Design review of the part built by this model. Coordinates are the model's own, in mm. A direction names the side the tool comes from. Coordinates: 2 decimals unless noted, no trailing zeros. Loops run counter-clockwise (first coordinate to the right, second up) from the corner with the lowest first, then second, coordinate; pieces in that order, holes last. Notation, with made-up numbers: (47.5, 46) - (59.5, 46) arc R17 ccw to (59.5, 56) - close; hole circle Ø9 at (82.25, 34.5). An arc over 180 degrees is marked (long way). Answer in a Markdown table with one row per item. Add a question column.
(1) Clearance check with flat-ended pins moving along their axes: pin 1 (0.8 mm diameter, centred on x = -4.5, z = 6.5, fed in from +Y); pin 2 (12 mm diameter, centred on y = 13, z = 15.5, fed in from +X); pin 3 (5.5 mm diameter, centred on y = 0, z = 5, fed in from -X). State where each tip first meets the part, or that it passes through.
(2) To check wall thickness, follow L1, parallel to Y at x = 0, z = 55.35; L2, parallel to X at y = -7, z = 55 (3 decimals); L3, parallel to Z at x = -3.5, y = -9.5. State the ranges of each line that lie inside material, in increasing order. Write a range as [from, to].
(3) For faces 5 (the face through (0, 4, 35)), 6 (the face through (6.428, 4.929, 23.493)), 7 (the face through (-5, 9, 54)), 8 (the face through (7.5, -1, 3)), list the 3-axis set-ups (+Z, -Z, +X, -X, +Y, -Y) from which the entire face can be reached by the end or side of a thin tool; tool diameter is ignored.
(4) We need section D-D, the plane y = 15. Write out the cut boundary in (x, z), plus the area to 3 significant figures.
(5) We need section B-B, the plane z = 5.5. Write out the cut boundary in (x, y).
(6) We need section C-C, the plane x = 0. Give the number of separate pieces and of enclosed holes in the cut face, plus the area to 3 significant figures.
(7) We need section A-A, the plane y = 0. Write out the cut boundary in (x, z), plus the area to 3 significant figures.
(8) The part is to be moulded in two halves that separate along Y. For faces 1 (the face through (-5, 4, 3)), 2 (the face through (-11.083, 8.101, 55.479)), 3 (the face through (-4.336, -19.524, 55.479)), 4 (the face through (0, -13, 55)), say which applies: released by +Y, released by -Y, zero draft, split by the parting line, or undercut.
from build123d import *

# Parameters (mm, degrees)
SKETCH_1_R               = 8.5
EXTRUDE_1_DEPTH          = 33
SKETCH_2_R               = 8.5
EXTRUDE_2_DEPTH          = 11
SKETCH_3_R               = 10
EXTRUDE_3_DEPTH          = 10
CHAMFER_2_SIZE           = 0.5
SKETCH_12_W              = 1
SKETCH_12_H              = 0.4
SKETCH_13_R              = 5
CUT_EXTRUDE_1_DEPTH      = 20
EXTRUDE_START            = 7.5
SKETCH_19_R              = 8.5
EXTRUDE_6_DEPTH          = 7.5
SKETCH_20_R              = 5
CUT_EXTRUDE_5_DEPTH      = 7.5
CUT_EXTRUDE_6_DEPTH      = 16.5
CUT_EXTRUDE_6_DEPTH_BACK = 16.5
SKETCH_21_R              = 1.5
SKETCH_14_R              = 20
SKETCH_14_R_2            = 2
EXTRUDE_7_DEPTH          = 3
EXTRUDE_START_2          = 7
SKETCH_23_R              = 5
EXTRUDE_8_DEPTH          = 7
CUT_EXTRUDE_START        = -44
SKETCH_24_R              = 5
CUT_EXTRUDE_7_DEPTH      = 44
SKETCH_31_R              = 7
SKETCH_31_R_2            = 5
EXTRUDE_10_DEPTH         = 20
EXTRUDE_11_DEPTH         = 84
SKETCH_33_R              = 1.5
CUT_EXTRUDE_8_DEPTH      = 26
EXTRUDE_START_3          = -3
SKETCH_35_R              = 13
SKETCH_35_R_2            = 7
EXTRUDE_12_DEPTH         = 3
SKETCH_36_R              = 1.5
CUT_EXTRUDE_10_DEPTH     = 3
CUT_EXTRUDE_START_2      = -20
SKETCH_38_R              = 20
CUT_EXTRUDE_12_DEPTH     = 20
SKETCH_39_W              = 15
SKETCH_39_H              = 6.010679791
CUT_EXTRUDE_13_DEPTH     = 20
SKETCH_40_W              = 3.690554248
SKETCH_40_H              = 8
SKETCH_40_W_2            = 3.213479815
CUT_EXTRUDE_14_DEPTH     = 20
SKETCH_42_W              = 19.43068456
SKETCH_42_H              = 3.441553847
CUT_EXTRUDE_16_DEPTH     = 20
CHAMFER_5_SIZE           = 1
CHAMFER_6_SIZE           = 1


with BuildPart() as part:
    # 草图1 → 凸台-拉伸1 (new body)
    with BuildSketch(Plane.XY):
        Circle(SKETCH_1_R)
    extrude(amount=EXTRUDE_1_DEPTH)

    # 草图2 → 凸台-拉伸2 (add)
    with BuildSketch(Plane.XY.offset(33)):
        Circle(SKETCH_2_R)
    extrude(amount=EXTRUDE_2_DEPTH)

    # 草图3 → 凸台-拉伸3 (add)
    with BuildSketch(Plane.XY.offset(44)):
        Circle(SKETCH_3_R)
    extrude(amount=EXTRUDE_3_DEPTH)

    # 倒角2
    chamfer_2_edges = [part.edges().sort_by_distance(p)[0] for p in [
        (-8.5, 0, 0),
    ]]
    chamfer(chamfer_2_edges, length=CHAMFER_2_SIZE)

    # 草图12 → 切除-旋转1 (revolve, cut)
    with BuildSketch(Plane(origin=(0, 0, 0), x_dir=(0, 0, -1), z_dir=(1, 0, 0)), mode=Mode.PRIVATE) as cut_revolve_1_sk:
        with Locations((-23.5, 8.3)):
            Rectangle(SKETCH_12_W, SKETCH_12_H)
    revolve(cut_revolve_1_sk.sketch.rotate(Axis((0, 0, 0), (0, 0, 1)), 90), axis=Axis((0, 0, 0), (0, 0, 1)), mode=Mode.SUBTRACT)

    # 草图13 → 切除-拉伸1 (cut)
    with BuildSketch(Plane(origin=(0, 0, 0), x_dir=(-1, 0, 0), z_dir=(0, 0, -1))):
        Circle(SKETCH_13_R)
    extrude(amount=-CUT_EXTRUDE_1_DEPTH, mode=Mode.SUBTRACT)

    # 草图19 → 凸台-拉伸6 (add)
    with BuildSketch(Plane(origin=(0, 0, 0.5), x_dir=(-1, 0, 0), z_dir=(0, 0, -1)).offset(EXTRUDE_START)):
        Circle(SKETCH_19_R)
    extrude(amount=-EXTRUDE_6_DEPTH)

    # 草图20 → 切除-拉伸5 (cut)
    with BuildSketch(Plane(origin=(0, 0, -7), x_dir=(-1, 0, 0), z_dir=(0, 0, -1))):
        Circle(SKETCH_20_R)
    extrude(amount=-CUT_EXTRUDE_5_DEPTH, mode=Mode.SUBTRACT)

    # 草图21 → 切除-拉伸6 (cut, two sides: drawn at the far end of the back side and taken through both)
    with BuildSketch(Plane(origin=(0, 0, 0), x_dir=(1, 0, 0), z_dir=(0, 1, 0)).offset(-CUT_EXTRUDE_6_DEPTH_BACK)):
        with Locations(Location((0, -3, 0), (0, 0, 90))):
            Circle(SKETCH_21_R)
    extrude(amount=CUT_EXTRUDE_6_DEPTH + CUT_EXTRUDE_6_DEPTH_BACK, mode=Mode.SUBTRACT)

    # 草图14 → 凸台-拉伸7 (add)
    with BuildSketch(Plane.XY.offset(54)):
        Circle(SKETCH_14_R)
        with Locations((0, 15)):
            Circle(SKETCH_14_R_2, mode=Mode.SUBTRACT)
        with Locations((12.990381057, 7.5)):
            Circle(SKETCH_14_R_2, mode=Mode.SUBTRACT)
        with Locations((12.990381057, -7.5)):
            Circle(SKETCH_14_R_2, mode=Mode.SUBTRACT)
        with Locations((0, -15)):
            Circle(SKETCH_14_R_2, mode=Mode.SUBTRACT)
        with Locations((-12.990381057, -7.5)):
            Circle(SKETCH_14_R_2, mode=Mode.SUBTRACT)
        with Locations((-12.990381057, 7.5)):
            Circle(SKETCH_14_R_2, mode=Mode.SUBTRACT)
    extrude(amount=EXTRUDE_7_DEPTH)

    # 草图23 → 凸台-拉伸8 (add)
    with BuildSketch(Plane(origin=(0, 0, 20), x_dir=(-1, 0, 0), z_dir=(0, 0, -1)).offset(EXTRUDE_START_2)):
        Circle(SKETCH_23_R)
    extrude(amount=-EXTRUDE_8_DEPTH)

    # 草图24 → 切除-拉伸7 (cut)
    with BuildSketch(Plane.XY.offset(57).offset(CUT_EXTRUDE_START)):
        with Locations(Location((0, 0, 0), (0, 0, 180))):
            Circle(SKETCH_24_R)
    extrude(amount=CUT_EXTRUDE_7_DEPTH, mode=Mode.SUBTRACT)

    # 草图31 → 凸台-拉伸10 (add)
    with BuildSketch(Plane.XY.offset(57)):
        Circle(SKETCH_31_R)
        with Locations(Location((0, 0, 0), (0, 0, 180))):
            Circle(SKETCH_31_R_2, mode=Mode.SUBTRACT)
    extrude(amount=EXTRUDE_10_DEPTH)

    # 草图32 → 凸台-拉伸11 (add)
    with BuildSketch(Plane(origin=(0, 0, -7), x_dir=(-1, 0, 0), z_dir=(0, 0, -1))):
        with BuildLine():
            Line((-3, 4), (3, 4))
            ThreePointArc((3, 4), (0, 5), (-3, 4))
        make_face()
    extrude(amount=-EXTRUDE_11_DEPTH)

    # 草图33 → 切除-拉伸8 (cut)
    with BuildSketch(Plane.XZ.offset(-4)):
        with Locations(Location((0, 3, 0), (0, 0, 270))):
            Circle(SKETCH_33_R)
    extrude(amount=-CUT_EXTRUDE_8_DEPTH, mode=Mode.SUBTRACT)

    # 草图35 → 凸台-拉伸12 (add)
    with BuildSketch(Plane.XY.offset(74).offset(EXTRUDE_START_3)):
        Circle(SKETCH_35_R)
        Circle(SKETCH_35_R_2, mode=Mode.SUBTRACT)
    extrude(amount=EXTRUDE_12_DEPTH)

    # 草图36 → 切除-拉伸10 (cut)
    with BuildSketch(Plane.XY.offset(74)):
        with Locations((0, 10)):
            Circle(SKETCH_36_R)
        with Locations((8.660254038, 5)):
            Circle(SKETCH_36_R)
        with Locations((8.660254038, -5)):
            Circle(SKETCH_36_R)
        with Locations((0, -10)):
            Circle(SKETCH_36_R)
        with Locations((-8.660254038, -5)):
            Circle(SKETCH_36_R)
        with Locations((-8.660254038, 5)):
            Circle(SKETCH_36_R)
    extrude(amount=-CUT_EXTRUDE_10_DEPTH, mode=Mode.SUBTRACT)

    # 草图38 → 切除-拉伸12 (cut)
    with BuildSketch(Plane.XY.offset(77).offset(CUT_EXTRUDE_START_2)):
        Circle(SKETCH_38_R)
    extrude(amount=CUT_EXTRUDE_12_DEPTH, mode=Mode.SUBTRACT)

    # 草图39 → 切除-拉伸13 (cut)
    with BuildSketch(Plane(origin=(0, 0, -7), x_dir=(-1, 0, 0), z_dir=(0, 0, -1))):
        with Locations((0, 7.005339896)):
            Rectangle(SKETCH_39_W, SKETCH_39_H)
    extrude(amount=-CUT_EXTRUDE_13_DEPTH, mode=Mode.SUBTRACT)

    # 草图40 → 切除-拉伸14 (cut)
    with BuildSketch(Plane(origin=(0, 0, -7), x_dir=(-1, 0, 0), z_dir=(0, 0, -1))):
        with Locations((-9.345277124, 0)):
            Rectangle(SKETCH_40_W, SKETCH_40_H)
        with Locations((9.106739908, 0)):
            Rectangle(SKETCH_40_W_2, SKETCH_40_H)
    extrude(amount=-CUT_EXTRUDE_14_DEPTH, mode=Mode.SUBTRACT)

    # 草图42 → 切除-拉伸16 (cut)
    with BuildSketch(Plane(origin=(0, 0, -7), x_dir=(-1, 0, 0), z_dir=(0, 0, -1))):
        with Locations((-0.246054433, -8.720776924)):
            Rectangle(SKETCH_42_W, SKETCH_42_H)
    extrude(amount=-CUT_EXTRUDE_16_DEPTH, mode=Mode.SUBTRACT)

    # 倒角5
    chamfer_5_edges = [part.edges().sort_by_distance(p)[0] for p in [
        (-7.5, 4, 3),
        (7.5, 4, 3),
    ]]
    chamfer(chamfer_5_edges, length=CHAMFER_5_SIZE)

    # 倒角6
    # the kernel refuses this chamfer: 1, 0.714285714 mm, written as the material it takes off along each edge
    with BuildSketch(Plane(origin=(-3, 4, -9.571682988), x_dir=(-1, 0, 0), z_dir=(0, 0, 1)), Plane(origin=(3, 4, 13), x_dir=(1, 0, 0), z_dir=(0, 0, -1))) as chamfer_6_piece_1:
        with BuildLine():
            Line((CHAMFER_6_SIZE, 0), (0.535533906, 0.464466094))
            ThreePointArc((0.535533906, 0.464466094), (0.274930492, 0.221795364), (0, 0))
            Line((0, 0), (CHAMFER_6_SIZE, 0))
        make_face()
    extrude(amount=22.571682988, mode=Mode.SUBTRACT)


solid = part.part
Responses:
| question | item | result |
|---|---|---|
| 1 | pin 1 | stops at y = 4 |
| 1 | pin 2 | stops at x = 4.82 |
| 1 | pin 3 | stops at x = -7.5 |
| 2 | L1 | y = [-20, -17], [-13, -5], [4, 13], [17, 20] |
| 2 | L2 | x = [-18.735, -14.927], [-11.054, 11.054], [14.927, 18.735] |
| 2 | L3 | z = [54, 57] |
| 3 | face 5 | +Z, -Z |
| 3 | face 6 | none |
| 3 | face 7 | -Z |
| 3 | face 8 | -Z, +X, +Y, -Y |
| 4 | outline | (-13.23, 54) - (-2, 54) - (-2, 57) - (-13.23, 57) - close; (2, 54) - (13.23, 54) - (13.23, 57) - (2, 57) - close |
| 4 | area | 67.4 mm2 |
| 5 | outline | (-7.5, -4) arc R8.5 ccw to (-4.82, -7) - (4.82, -7) arc R8.5 ccw to (7.5, -4) - (7.5, 3) - (6.5, 4) - (4, 4) - (3.54, 3.54) arc R5 cw (long way) to (-3.54, 3.54) - (-4, 4) - (-6.5, 4) - (-7.5, 3) - close |
| 6 | separate pieces | 5 |
| 6 | enclosed holes | 0 |
| 6 | area | 460 mm2 |
| 7 | outline | (-20, 54) - (-10, 54) - (-10, 44) - (-8.5, 44) - (-8.5, 24) - (-8.1, 24) - (-8.1, 23) - (-8.5, 23) - (-8.5, 13) - (-7.5, 13) - (-7.5, -7) - (-5, -7) - (-5, 57) - (-20, 57) - close; (5, -7) - (7.5, -7) - (7.5, 13) - (8.5, 13) - (8.5, 23) - (8.1, 23) - (8.1, 24) - (8.5, 24) - (8.5, 44) - (10, 44) - (10, 54) - (20, 54) - (20, 57) - (5, 57) - close |
| 7 | area | 506 mm2 |
| 8 | face 1 | released by +Y |
| 8 | face 2 | undercut |
| 8 | face 3 | split by the parting line |
| 8 | face 4 | undercut |
